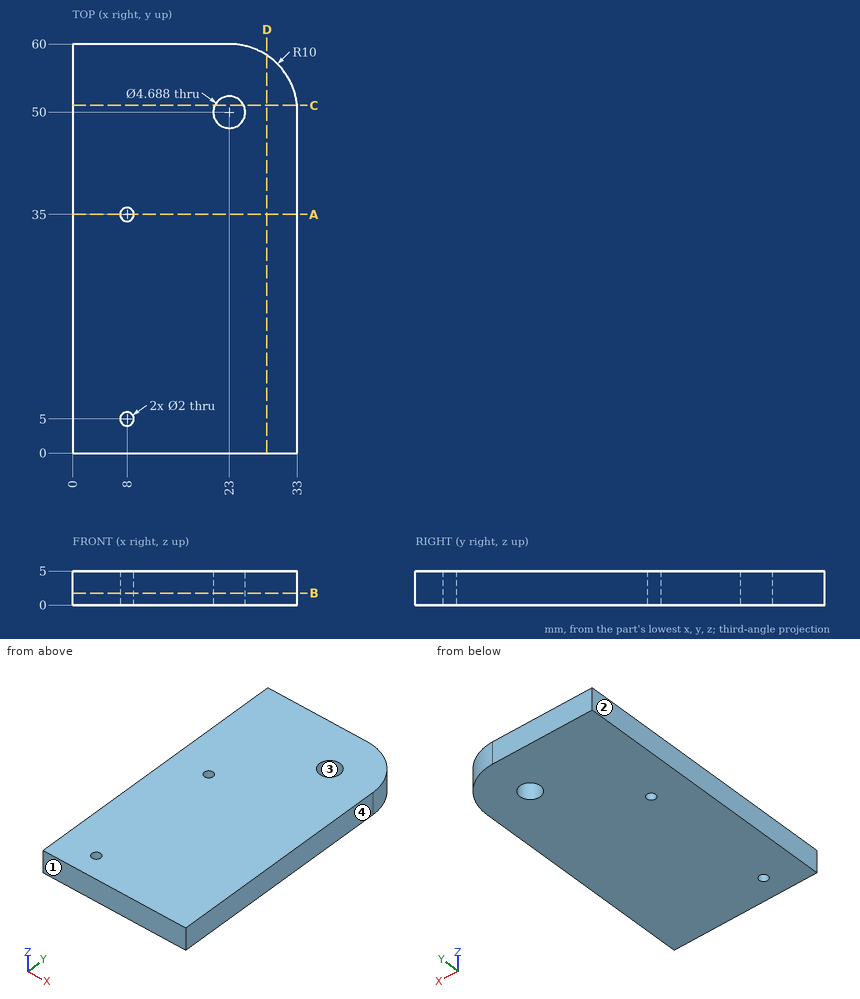
The drawing under review shows one solid part. Ordinate dimensions are in mm from its lowest x, y, z. Coordinates: 2 decimals unless noted, no trailing zeros. Loops run counter-clockwise (first coordinate to the right, second up) from the corner with the lowest first, then second, coordinate; pieces in that order, holes last. Notation, with made-up numbers: (-17, -29) - (-11, -29) arc R11 ccw to (-11, -18) - close; hole circle Ø8 at (1, 36.25). An arc over 180 degrees is marked (long way). Return JSON: item names as keys, results as strings.
Item 1: Take a section at D-D (x = 28.5). Give the boundary of the cut face in (y, z).
Determined:
{"outline": "(0, 0) - (58.35, 0) - (58.35, 5) - (0, 5) - close"}
Item 2: For line 1 (Y direction, x = 8, z = 3.1); line 2 (Y direction, x = 23, z = 3.05); line 3 (X direction, y = 4.5, z = 4.1) (1 decimal), list the stretches that pass through material, from the lowest coordinate up.
Determined:
{"line 1": "y = 0 to 4, 6 to 34, 36 to 60", "line 2": "y = 0 to 47.66, 52.34 to 60", "line 3": "x = 0 to 7.1, 8.9 to 33"}
Item 3: Take a section at B-B (z = 1.75). Give the boundary of the cut face in (x, y).
Determined:
{"outline": "(0, 0) - (33, 0) - (33, 50) arc R10 ccw to (23, 60) - (0, 60) - close; hole circle Ø2 at (8, 5); hole circle Ø2 at (8, 35); hole circle Ø4.69 at (23, 50)"}
Item 4: Take a section at C-C (y = 51). Give the boundary of the cut face in (x, z).
Determined:
{"outline": "(0, 0) - (20.88, 0) - (20.88, 5) - (0, 5) - close; (25.12, 0) - (32.95, 0) - (32.95, 5) - (25.12, 5) - close"}
Item 5: Take a section at A-A (y = 35). Give the boundary of the cut face in (x, z).
Determined:
{"outline": "(0, 0) - (7, 0) - (7, 5) - (0, 5) - close; (9, 0) - (33, 0) - (33, 5) - (9, 5) - close"}
Item 6: Mouldability with a two-part tool opening along X and no side actions: class the marked faces 1, 2, 3 and 4 as pulls with the +X half, pulls with the -X half, needs draft (parallel to the pull), parting line crosses it, or undercut.
Determined:
{"face 1": "needs draft", "face 2": "pulls with the -X half", "face 3": "undercut", "face 4": "pulls with the +X half"}
